Verification items for the finished model (mm, model axes). Face numbers are marked on the shaded views. A direction names the side the tool comes from. Give positions to 0.01 mm unless a question says otherwise; leave off trailing zeros. Order: outer loops, then holes, each group sorted by start corner. A loop starts at its lowest first (then second) coordinate and runs counter-clockwise, first axis right, second up. Notation, with made-up numbers: (-29.75, 84.5) -> (-8.75, 84.5) arc R20 cw to (-8.75, 116.5) -> close; hole circle Ø2 at (-20, 14). An arc over 180 degrees is marked (long way). One line per question, with ' | ' between items. Start each with the question number.
Q1. Section check B-B on z = 1.75. Record the cut outline in (x, y) (3 decimals).
Q2. Section check A-A on z = 9.25. Record the cut outline in (x, y) (3 decimals).
Q3. Material ranges on probe 1 along Y at (x, z) = (40.4, 3.25) (3 decimals); probe 2 along Y at (x, z) = (40.4, 8.75) (3 decimals); probe 3 along Z at (x, y) = (42, -19.5), recorded low to high. Write a range as [from, to].
Q4. Go/stop test with flat-tipped pins: pin 1 (1.5 mm diameter, centred on y = -21, z = 5, fed in from -X); pin 2 (6 mm diameter, centred on y = -29.5, z = 9, fed in from -X); pin 3 (2.5 mm diameter, centred on x = 40.4, y = -23.75, fed in from +Z); pin 4 (12 mm diameter, centred on y = -24, z = -3.5, fed in from +X). Record where each tip stops, or that it passes through.
Q5. Mould release check, pull along X, two halves, no side actions. Record for the marked faces 3, 4 and 5: released by +X, released by -X, zero draft, split by the parting line, or undercut.
Q6. Access from +Z, -Z, +X, -X, +Y, -Y to the whole of each face (thin tool, end or side, straight path). Record for the marked faces 1 and 2.
from build123d import *

# Parameters (mm, degrees)
SKETCH1_R               = 3.873
BOSS_EXTRUDE1_DEPTH     = 7
FILLET1_R               = 2.000000064
BOSS_EXTRUDE2_START     = 3
SKETCH2_R               = 8
SKETCH2_R_2             = 3.873
BOSS_EXTRUDE2_DEPTH     = 3
SKETCH3_R               = 13
BOSS_EXTRUDE3_DEPTH     = 2.5
CHAMFER1_SIZE           = 5.196152423
CHAMFER1_SIZE_2         = 3
BOSS_EXTRUDE4_START     = 8
SKETCH4_R               = 3.873
SKETCH4_R_2             = 1.435
BOSS_EXTRUDE4_DEPTH     = 8
BOSS_EXTRUDE5_START     = 0.5
SKETCH4_3_R             = 5.5
SKETCH4_3_R_2           = 3.873
SKETCH4_3_R_3           = 1.435
BOSS_EXTRUDE5_DEPTH     = 0.5
CUT_EXTRUDE1_DEPTH      = 67.017971016
CUT_EXTRUDE1_DEPTH_BACK = 67.017971016
SKETCH6_R               = 1.435


with BuildPart() as part:
    # Sketch1 → Boss-Extrude1 (new body)
    with BuildSketch(Plane.XY):
        with Locations((40.399999972, -23.75)):
            Circle(SKETCH1_R)
    extrude(amount=-BOSS_EXTRUDE1_DEPTH)

    # Fillet1
    fillet1_edges = [part.edges().sort_by_distance(p)[0] for p in [
        (36.526999972, -23.75, -7),
    ]]
    fillet(fillet1_edges, radius=FILLET1_R)

    # Sketch2 → Boss-Extrude2 (add)
    # profile 1 of 2: a face of its own
    with BuildSketch(Plane.XY.offset(BOSS_EXTRUDE2_START)):
        with Locations((40.399999972, -23.75)):
            Circle(SKETCH2_R)
        with Locations((40.399999972, -23.75)):
            Circle(SKETCH2_R_2, mode=Mode.SUBTRACT)
    # profile 2 of 2: a face of its own
    with BuildSketch(Plane.XY.offset(BOSS_EXTRUDE2_START)):
        with Locations((40.399999972, -23.75)):
            Circle(SKETCH2_R_2)
    extrude(amount=-BOSS_EXTRUDE2_DEPTH)

    # Sketch3 → Boss-Extrude3 (add)
    with BuildSketch(Plane.XY.offset(3)):
        with Locations(Location((40.399999972, -23.75, 0), (0, 0, 180))):
            Circle(SKETCH3_R)
    extrude(amount=BOSS_EXTRUDE3_DEPTH)

    # Chamfer1
    # the kernel refuses this chamfer: 5.196152423, 3 mm, written as the material it adds along each edge
    with BuildSketch(Plane(origin=(40.399999972, -23.75, 3), x_dir=(1, 0, 0), z_dir=(0, -1, 0))) as chamfer1_piece_1_section:
        Polygon((8 + CHAMFER1_SIZE, 0), (8, -CHAMFER1_SIZE_2), (8, 0), align=None)
    chamfer1_piece_1 = revolve(axis=Axis((40.399999972, -23.75, 3), (0, 0, 1)), mode=Mode.PRIVATE)
    chamfer1_piece_1 = chamfer1_piece_1 & Plane(origin=(40.399999972, -23.75, 1.510979696), x_dir=(-1, 0, 0), z_dir=(0, 0, -1)) * Cylinder(13, 53, mode=Mode.PRIVATE)
    add(chamfer1_piece_1)

    # Sketch4 → Boss-Extrude4 (add)
    with BuildSketch(Plane.XY.offset(5.5).offset(BOSS_EXTRUDE4_START)):
        with Locations((40.399999972, -23.75)):
            Circle(SKETCH4_R)
        with Locations(Location((40.399999972, -23.75, 0), (0, 0, 180))):
            Circle(SKETCH4_R_2, mode=Mode.SUBTRACT)
    extrude(amount=-BOSS_EXTRUDE4_DEPTH)

    # Sketch4<3> → Boss-Extrude5 (add)
    # profile 1 of 2: a face of its own
    with BuildSketch(Plane.XY.offset(5.5).offset(BOSS_EXTRUDE5_START)):
        with Locations(Location((40.399999972, -23.75, 0), (0, 0, 180))):
            Circle(SKETCH4_3_R)
        with Locations((40.399999972, -23.75)):
            Circle(SKETCH4_3_R_2, mode=Mode.SUBTRACT)
    # profile 2 of 2: a face of its own
    with BuildSketch(Plane.XY.offset(5.5).offset(BOSS_EXTRUDE5_START)):
        with Locations((40.399999972, -23.75)):
            Circle(SKETCH4_3_R_2)
        with Locations(Location((40.399999972, -23.75, 0), (0, 0, 180))):
            Circle(SKETCH4_3_R_3, mode=Mode.SUBTRACT)
    extrude(amount=-BOSS_EXTRUDE5_DEPTH)

    # Sketch6 → Cut-Extrude1 (cut, two sides: drawn at the far end of the back side and taken through both)
    with BuildSketch(Plane.XY.offset(5.5).offset(-CUT_EXTRUDE1_DEPTH_BACK)):
        with Locations(Location((40.399999972, -23.75, 0), (0, 0, 180))):
            Circle(SKETCH6_R)
    extrude(amount=CUT_EXTRUDE1_DEPTH + CUT_EXTRUDE1_DEPTH_BACK, mode=Mode.SUBTRACT)


solid = part.part
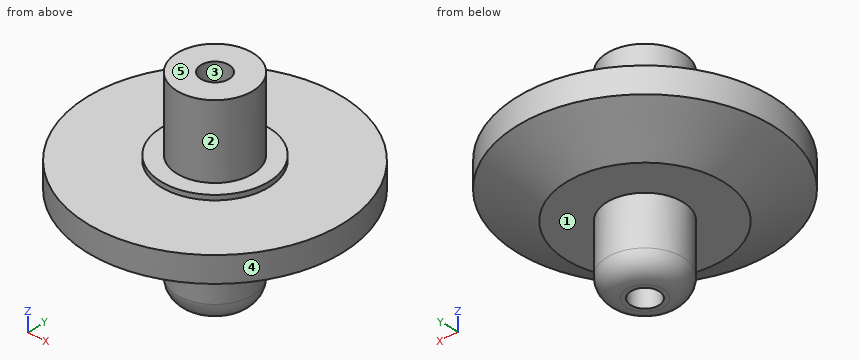
Filled in:
1) outline: circle Ø22.062 at (40.4, -23.75); hole circle Ø2.87 at (40.4, -23.75)
2) outline: circle Ø7.746 at (40.4, -23.75); hole circle Ø2.87 at (40.4, -23.75)
3) probe 1: [-36.75, -25.185], [-22.315, -10.75] | probe 2: [-27.623, -25.185], [-22.315, -19.877] | probe 3: [0, 6]
4) pin 1: x = 27.55 | pin 2: x = 37.67 | pin 3: through | pin 4: x = 52.73
5) face 3: undercut | face 4: split by the parting line | face 5: zero draft
6) face 1: -Z | face 2: +Z
